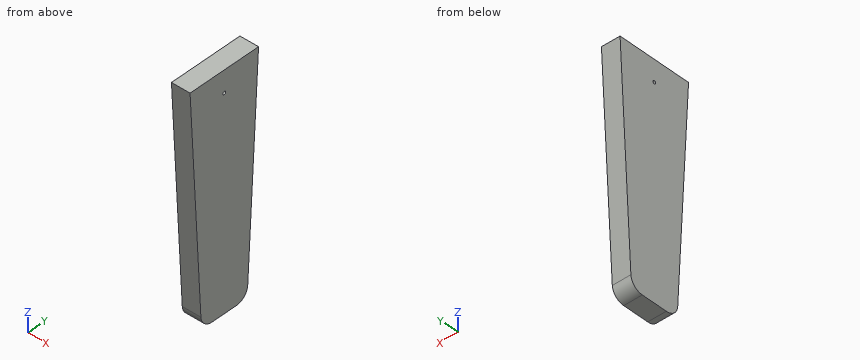
from build123d import *

# Parameters (mm, degrees)
F0_R     = 1.5875
F1_DEPTH = 19.05


with BuildPart() as f1:
    # F0 (on Right) → F1 (new body)
    with BuildSketch(Plane.YZ):
        with BuildLine():
            ThreePointArc((-42.08502, -102.493227), (-38.138072, -111.027168), (-29.403534, -114.507741))
            Line((-29.403534, -114.507741), (-2.667641, -114.507741))
            ThreePointArc((-2.667641, -114.507741), (6.066898, -111.027168), (10.013846, -102.493227))
            Line((10.013846, -102.493227), (22.064413, 120.442259))
            Line((22.064413, 120.442259), (-54.135587, 120.442259))
            Line((-54.135587, 120.442259), (-42.08502, -102.493227))
        make_face()
        with Locations((-16.035587, 98.217259)):
            Circle(F0_R, mode=Mode.SUBTRACT)
    extrude(amount=F1_DEPTH)


solid = f1.part
CAD build for the part. Positions are in the model's coordinates, mm. Give positions to 0.01 mm unless a question says otherwise; leave off trailing zeros. Loops run counter-clockwise (first coordinate to the right, second up) from the corner with the lowest first, then second, coordinate; pieces in that order, holes last. Notation, with made-up numbers: M 46.25,-18 L 67.25,-18 A20 cw 67.25,-5 Z; hole C 23,14.25 d2. An arc over 180 degrees is marked long. Write each question's results on one line, items separated by ' | '.
Q1. Band-saw the part on C-C on y = -48.5. Write the cut outline in (x, z), and give its area (3 significant figures).
Geometry check:
outline: M 0,16.18 L 19.05,16.18 L 19.05,120.44 L 0,120.44 Z | area: 1,990 mm²
Q2. Band-saw the part on B-B on z = -33.5. Write the cut outline in (x, y), and give its area (3 significant figures).
Geometry check:
outline: M 0,-45.81 L 19.05,-45.81 L 19.05,13.74 L 0,13.74 Z | area: 1,130 mm²
Q3. Band-saw the part on A-A on x = 8.5. Write the cut outline in (y, z) (1 decimal).
Geometry check:
outline: M -54.1,120.4 L -42.1,-102.5 A12.7 ccw -29.4,-114.5 L -2.7,-114.5 A12.7 ccw 10,-102.5 L 22.1,120.4 Z; hole C -16,98.2 d3.2
Q4. Probe probe 1 along Z at (x, y) = (1.5, -35); probe 2 along Z at (x, y) = (11.75, -31); probe 3 along Y at (x, z) = (9.5, -90). List the from-to ranges inside material, lowest first.
Geometry check:
probe 1: z = -113.21 to 120.44 | probe 2: z = -114.41 to 120.44 | probe 3: y = -42.76 to 10.69
Q5. Flat gauge pins, fed straight in: P1, Ø1, axis at x = 7, z = -33.5, coming from the -Y side; P2, Ø3, axis at x = 11, z = -88.5, coming from the -Y side; P3, Ø4, axis at x = 17, z = 81.5, coming from the -Y side. Where does each tip first touch, or does it go through?
Geometry check:
P1: stops at y = -45.84 | P2: stops at y = -42.92 | P3: stops at y = -52.14
